Check sheet for the modelled part. Datum: model origin and axes. Units: mm. A direction names the side the tool comes from. Round coordinates to 2 decimals unless told otherwise and drop trailing zeros. Order: outer loops, then holes, each group sorted by start corner. A loop starts at its lowest first (then second) coordinate and runs counter-clockwise, first axis right, second up.
Q1. Cross-section at C-C on y = 75. Record the cut outline in (x, z), then the cut area to 3 significant figures.
Q2. Cross-section at B-B on z = 0. Record the cut outline in (x, y).
Q3. Set-up check for faces 1 (the cylindrical face through (19.51, 84.915, 1.302)), 2 (the flat face through (30, -75, 0)), 3 (the flat face through (27, 55, 0)): record each of +Z, -Z, +X, -X, +Y, -Y from which the full face is reachable in a straight line by a thin tool's end or side.
Q4. Cross-section at D-D on z = -22. Record the cut outline in (x, y).
Q5. Depth check by flat-ended pin: P1, Ø4, axis at y = -55.5, z = 5.5, coming from the +X side; P2, Ø5, axis at y = -5, z = -10, coming from the +X side; P3, Ø12, axis at x = 46, z = -8, coming from the -Y side. Enter the tip coordinate at first touch or a pass-through.
Q6. Mould release check, pull along Y, two halves, no side actions. Record for faces 4 (the flat face through (15, -55, 0)), 5 (the flat face through (7, -95, 0)), 6 (the flat face through (-15, 1, 0)), 7 (the flat face through (0, 1, 0)): +Y half, -Y half, draft (parallel to the pull), parting line (faces both ways), or undercut.
Q7. Scan lines: probe 1 along Y at (x, z) = (26, 0); probe 2 along Y at (x, z) = (-0.5, 0); probe 3 along Y at (x, z) = (35.5, 0). Record each from-to range of solid material in increasing order.
Q8. Cross-section at A-A on x = 5. Record the cut outline in (y, z).
from build123d import *

# Parameters (mm, degrees)
SKETCH1_W           = 50
SKETCH1_H           = 40
SKETCH1_R           = 10
BOSS_EXTRUDE1_DEPTH = 55
BOSS_EXTRUDE2_START = -15
SKETCH1_3_W         = 50
SKETCH1_3_H         = 190
SKETCH1_3_R         = 10
BOSS_EXTRUDE2_DEPTH = 15
SKETCH1_4_W         = 50
SKETCH1_4_H         = 40
BOSS_EXTRUDE3_DEPTH = 30


with BuildPart() as part:
    # Sketch1 → Boss-Extrude1 (new body)
    with BuildSketch(Plane(origin=(0, 0, 0), x_dir=(0, 0, -1), z_dir=(1, 0, 0))):
        with Locations((0, 75)):
            Rectangle(SKETCH1_W, SKETCH1_H)
        with Locations((0, 75)):
            Circle(SKETCH1_R, mode=Mode.SUBTRACT)
    extrude(amount=BOSS_EXTRUDE1_DEPTH)

    # Sketch1<3> → Boss-Extrude2 (add)
    with BuildSketch(Plane(origin=(0, 0, 0), x_dir=(0, 0, -1), z_dir=(1, 0, 0)).offset(BOSS_EXTRUDE2_START)):
        Rectangle(SKETCH1_3_W, SKETCH1_3_H)
        with Locations((0, 75)):
            Circle(SKETCH1_3_R, mode=Mode.SUBTRACT)
    extrude(amount=BOSS_EXTRUDE2_DEPTH)

    # Sketch1<4> → Boss-Extrude3 (add)
    with BuildSketch(Plane(origin=(0, 0, 0), x_dir=(0, 0, -1), z_dir=(1, 0, 0))):
        with Locations((0, -75)):
            Rectangle(SKETCH1_4_W, SKETCH1_4_H)
    extrude(amount=BOSS_EXTRUDE3_DEPTH)


solid = part.part
Results found:
1. outline: (-15, -25) - (55, -25) - (55, -10) - (-15, -10) - close; (-15, 10) - (55, 10) - (55, 25) - (-15, 25) - close
1. area: 2,100 mm2
2. outline: (-15, -95) - (30, -95) - (30, -55) - (0, -55) - (0, 55) - (55, 55) - (55, 65) - (-15, 65) - close; (-15, 85) - (55, 85) - (55, 95) - (-15, 95) - close
3. face 1: +X, -X
3. face 2: +Z, -Z, +X, -Y
3. face 3: +Z, -Z, +X
4. outline: (-15, -95) - (30, -95) - (30, -55) - (0, -55) - (0, 55) - (55, 55) - (55, 95) - (-15, 95) - close
5. P1: stops at x = 30
5. P2: stops at x = 0
5. P3: stops at y = 55
6. face 4: undercut
6. face 5: -Y half
6. face 6: draft
6. face 7: undercut
7. probe 1: y = -95 to -55, 55 to 65, 85 to 95
7. probe 2: y = -95 to 65, 85 to 95
7. probe 3: y = 55 to 65, 85 to 95
8. outline: (-95, -25) - (-55, -25) - (-55, 25) - (-95, 25) - close; (55, -25) - (95, -25) - (95, 25) - (55, 25) - close; hole circle Ø20 at (75, 0)
